```python
from build123d import *

# Parameters (mm, degrees)
F0_W     = 20.9161378443
F0_H     = 9.225605987
F1_DEPTH = 2.54
F0_H_2   = 32.3809729889
F2_DEPTH = 15.748
F4_DEPTH = 25.4
F5_DEPTH = 1.8034


with BuildPart() as f1:
    # F0 (on Top) → F1 (new body)
    with BuildSketch(Plane.XY):
        with BuildLine():
            ThreePointArc((-10.4580689222, -20.803289488), (0, -31.2613584101), (10.4580689222, -20.803289488))
            Line((10.4580689222, -20.803289488), (-10.4580689222, -20.803289488))
        make_face()
        with Locations((0, -16.1904864945)):
            Rectangle(F0_W, F0_H)
    extrude(amount=F1_DEPTH)

    # F0 (on Top) → F2 (join)
    with BuildSketch(Plane.XY):
        with Locations((0, 4.6128029935)):
            Rectangle(F0_W, F0_H_2)
    extrude(amount=F2_DEPTH)

    # F3 (on face) → F4 (cut)
    with BuildSketch(Plane(origin=(-10.4580689222, 0, 0), x_dir=(0, -1, 0), z_dir=(-1, 0, 0))):
        with BuildLine():
            Line((-4.6128029935, 4.7834570753), (-4.6128029935, 7.874))
            Line((-4.6128029935, 7.874), (-7.7033459182, 7.874))
            ThreePointArc((-7.7033459182, 7.874), (-6.7981468531, 5.6886561404), (-4.6128029935, 4.7834570753))
        make_face()
        with BuildLine():
            Line((-1.5222600688, 7.874), (-4.6128029935, 7.874))
            Line((-4.6128029935, 7.874), (-4.6128029935, 4.7834570753))
            ThreePointArc((-4.6128029935, 4.7834570753), (-2.4274591339, 5.6886561404), (-1.5222600688, 7.874))
        make_face()
        with BuildLine():
            ThreePointArc((-1.5222600688, 7.874), (-2.4274591339, 10.0593438596), (-4.6128029935, 10.9645429247))
            Line((-4.6128029935, 10.9645429247), (-4.6128029935, 7.874))
            Line((-4.6128029935, 7.874), (-1.5222600688, 7.874))
        make_face()
        with BuildLine():
            Line((-4.6128029935, 7.874), (-4.6128029935, 10.9645429247))
            ThreePointArc((-4.6128029935, 10.9645429247), (-6.7981468531, 10.0593438596), (-7.7033459182, 7.874))
            Line((-7.7033459182, 7.874), (-4.6128029935, 7.874))
        make_face()
    extrude(amount=-F4_DEPTH, mode=Mode.SUBTRACT)

    # F3 (on face) → F5 (cut)
    with BuildSketch(Plane(origin=(-10.4580689222, 0, 0), x_dir=(0, -1, 0), z_dir=(-1, 0, 0))):
        with BuildLine():
            Line((-4.6128029935, 10.9645429247), (-4.6128029935, 13.1498547085))
            ThreePointArc((-4.6128029935, 13.1498547085), (-8.3433956344, 11.6045926409), (-9.888657702, 7.874))
            Line((-9.888657702, 7.874), (-7.7033459182, 7.874))
            ThreePointArc((-7.7033459182, 7.874), (-6.7981468531, 10.0593438596), (-4.6128029935, 10.9645429247))
        make_face()
        with BuildLine():
            ThreePointArc((0.663051715, 7.874), (-0.8822103526, 11.6045926409), (-4.6128029935, 13.1498547085))
            Line((-4.6128029935, 13.1498547085), (-4.6128029935, 10.9645429247))
            ThreePointArc((-4.6128029935, 10.9645429247), (-2.4274591339, 10.0593438596), (-1.5222600688, 7.874))
            Line((-1.5222600688, 7.874), (0.663051715, 7.874))
        make_face()
        with BuildLine():
            ThreePointArc((-4.6128029935, 2.5981452915), (-0.8822103526, 4.1434073591), (0.663051715, 7.874))
            Line((0.663051715, 7.874), (-1.5222600688, 7.874))
            ThreePointArc((-1.5222600688, 7.874), (-2.4274591339, 5.6886561404), (-4.6128029935, 4.7834570753))
            Line((-4.6128029935, 4.7834570753), (-4.6128029935, 2.5981452915))
        make_face()
        with BuildLine():
            Line((-7.7033459182, 7.874), (-9.888657702, 7.874))
            ThreePointArc((-9.888657702, 7.874), (-8.3433956344, 4.1434073591), (-4.6128029935, 2.5981452915))
            Line((-4.6128029935, 2.5981452915), (-4.6128029935, 4.7834570753))
            ThreePointArc((-4.6128029935, 4.7834570753), (-6.7981468531, 5.6886561404), (-7.7033459182, 7.874))
        make_face()
    extrude(amount=-F5_DEPTH, mode=Mode.SUBTRACT)


solid = f1.part
```
Build history of the part. All positions in model axes, mm. A direction names the side the tool comes from. Give positions to 0.01 mm unless a question says otherwise; leave off trailing zeros. Order: outer loops, then holes, each group sorted by start corner. A loop starts at its lowest first (then second) coordinate and runs counter-clockwise, first axis right, second up. Notation, with made-up numbers: M -14,33 L 40,33 A17 ccw 40,39 Z; hole C 9,12 d9. An arc over 180 degrees is marked long. Return JSON: item names as keys, results as strings.
Q1. Band-saw the part on D-D (y = -14.5). Give the cut face in (x, z), then the cut area to 3 significant figures.
Answer list:
{"outline": "M -10.46,0 L 10.46,0 L 10.46,2.54 L -10.46,2.54 Z", "area": "53.1 mm^2"}
Q2. Flat gauge pins, fed straight in: pin 1 (4 mm diameter, centred on x = -3.5, z = 8.5, fed in from -Y); pin 2 (6 mm diameter, centred on x = -0.5, y = -22, fed in from +Z). Where does each tip first touch, or does it go through?
Answer list:
{"pin 1": "stops at y = -11.58", "pin 2": "stops at z = 2.54"}
Q3. Two-plate mould, pull along Y, no slides. Class faces 3 (the face through (0, 20.803, 8)), 4 (the face through (0, 5, 15.748)), 5 (the face through (-8.655, 2.3, 5.6)): pulls with the +Y half, pulls with the -Y half, needs draft (parallel to the pull), parting line crosses it, or undercut.
Answer list:
{"face 3": "pulls with the +Y half", "face 4": "needs draft", "face 5": "undercut"}
Q4. 3-axis set-ups, long thin cutter, end or side, ignore diameter. For faces 1 (the face through (0, -11.578, 9)), 2 (the face through (-0.23, -31.26, 1.25)): which of +Z, -Z, +X, -X, +Y, -Y reach the whole face in a straight line?
Answer list:
{"face 1": "+Z, +X, -X, -Y", "face 2": "+Z, -Z, -Y"}
Q5. Wall check: probe 1 along Y at (x, z) = (-5.25, 8); probe 2 along Z at (x, y) = (-5.5, -14.5); probe 3 along Y at (x, z) = (-4.5, 11.5). Give the ranges that are in metal, low to high. Write a range as from..to.
Answer list:
{"probe 1": "y = -11.58..1.52, 7.7..20.8", "probe 2": "z = 0..2.54", "probe 3": "y = -11.58..20.8"}
Q6. Band-saw the part on C-C (y = 6.5). Give the cut face in (x, z).
Answer list:
{"outline": "M -10.46,0 L 10.46,0 L 10.46,5.43 L -8.65,5.43 L -8.65,2.95 L -10.46,2.95 Z; M -10.46,12.8 L -8.65,12.8 L -8.65,10.32 L 10.46,10.32 L 10.46,15.75 L -10.46,15.75 Z"}
Q7. Band-saw the part on B-B (z = 7.25). Give the cut face in (x, y).
Answer list:
{"outline": "M -10.46,-11.58 L 10.46,-11.58 L 10.46,1.59 L -8.65,1.59 L -8.65,-0.63 L -10.46,-0.63 Z; M -10.46,9.85 L -8.65,9.85 L -8.65,7.64 L 10.46,7.64 L 10.46,20.8 L -10.46,20.8 Z"}
Q8. Band-saw the part on A-A (x = 0). Give the cut face in (y, z), then the cut area to 3 significant figures.
Answer list:
{"outline": "M -31.26,0 L 20.8,0 L 20.8,15.75 L -11.58,15.75 L -11.58,2.54 L -31.26,2.54 Z; hole C 4.61,7.87 d6.18", "area": "530 mm^2"}
